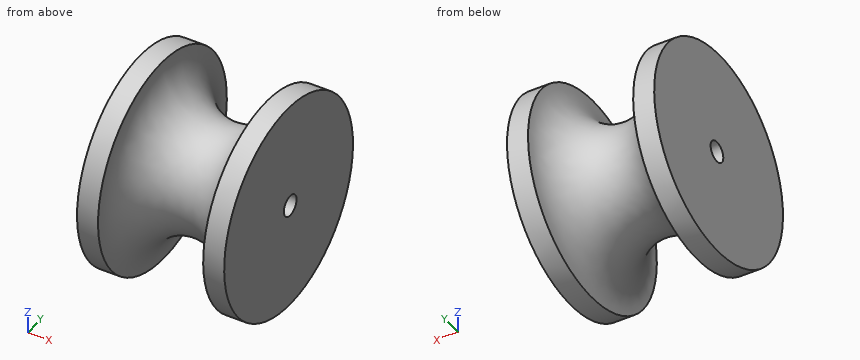
from build123d import *

# Parameters (mm, degrees)
F_97_0_0059_DIAMETER_HOLE2_D = 0.14986
SKETCH5_R                    = 2.5
CUT_EXTRUDE2_DEPTH           = 35.56


with BuildPart() as part:
    # Sketch1 → Revolve1 (revolve)
    with BuildSketch(Plane.XY, mode=Mode.PRIVATE) as revolve1_sk:
        with BuildLine():
            Line((-55.768127135, -1.934587814), (-50.688127135, -1.934587814))
            ThreePointArc((-50.688127135, -1.934587814), (-37.988127135, -14.634587814), (-25.288127135, -1.934587814))
            Line((-25.288127135, -1.934587814), (-20.208127135, -1.934587814))
            Line((-20.208127135, -1.934587814), (-20.208127135, -27.334587814))
            Line((-20.208127135, -27.334587814), (-55.768127135, -27.334587814))
            Line((-55.768127135, -27.334587814), (-55.768127135, -1.934587814))
        make_face()
    revolve(revolve1_sk.sketch.rotate(Axis((-55.768127135, -27.334587814, 0), (1, 0, 0)), 90), axis=Axis((-55.768127135, -27.334587814, 0), (1, 0, 0)))

    # #97 (0.0059) Diameter Hole2 (through all)
    with Locations(Plane.ZY.offset(55.768127135)):
        with Locations((0, -26.686562296)):
            Hole(F_97_0_0059_DIAMETER_HOLE2_D / 2)

    # Sketch5 → Cut-Extrude2 (cut)
    with BuildSketch(Plane.ZY.offset(55.768127135)):
        with Locations((-0.07493, -26.686562296)):
            Circle(SKETCH5_R)
    extrude(amount=-CUT_EXTRUDE2_DEPTH, mode=Mode.SUBTRACT)


solid = part.part
Input: part model. Units: mm. Frame: model coordinates. Give positions to 0.01 mm unless a question says otherwise; leave off trailing zeros. Loops run counter-clockwise (first coordinate to the right, second up) from the corner with the lowest first, then second, coordinate; pieces in that order, holes last. Notation, with made-up numbers: (-8, 60.5) -> (19, 60.5) arc R19 ccw to (19, 67.5) -> close; hole circle Ø4 at (-38.5, 42). An arc over 180 degrees is marked (long way). Answer as a JSON object with one key per item and string values. Group by question number.
Item 1: Cut plane B-B, the plane x = -24.5. Return the cut outline in (y, z), and give its area (3 significant figures).
Item 2: Cut plane C-C, the plane x = -48. Return the cut outline in (y, z).
Item 3: Line query: probe 1 along X at (y, z) = (-5.5, -12); probe 2 along X at (y, z) = (-10, -16.5); probe 3 along Z at (x, y) = (-45, -24.5). Output: solid intervals per line, ascending.
Item 4: Pin query (flat end, axial travel): P1, Ø1.5, axis at x = -50.5, y = -35.5, coming from the -Z side; P2, Ø8, axis at x = -34.5, z = 4, coming from the +Y side; P3, Ø1, axis at x = -35, y = -18, coming from the -Z side. Return the tip coordinate at first contact, or that it passes through.
Item 5: Cut plane A-A, the plane z = 0. Return the cut outline in (x, y).
Checks:
{
 "1": {"outline": "circle Ø50.8 at (-27.33, 0); hole circle Ø5 at (-26.69, -0.07)", "area": "2,010 mm²"},
 "2": {"outline": "circle Ø35.17 at (-27.33, 0); hole circle Ø5 at (-26.69, -0.07)"},
 "3": {"probe 1": "x = -55.77 to -50.68, -25.3 to -20.21", "probe 2": "x = -55.77 to -50.6, -25.37 to -20.21", "probe 3": "z = -14.54 to -1.29, 1.14 to 14.54"},
 "4": {"P1": "stops at z = -24.29", "P2": "stops at y = -12.59", "P3": "stops at z = -9.64"},
 "5": {"outline": "(-55.77, -52.73) -> (-50.69, -52.73) arc R12.7 cw to (-25.29, -52.73) -> (-20.21, -52.73) -> (-20.21, -29.19) -> (-55.77, -29.19) -> close; (-55.77, -24.19) -> (-20.21, -24.19) -> (-20.21, -1.93) -> (-25.29, -1.93) arc R12.7 cw to (-50.69, -1.93) -> (-55.77, -1.93) -> close"}
}
